from build123d import *

# Parameters (mm, degrees)
F0_W     = 20.141244
F0_H     = 20.141244
F0_R     = 8
F1_DEPTH = 5
F0_R_2   = 6.15
F2_DEPTH = 40
F3_DEPTH = 3


with BuildPart() as f1:
    # F0 (on Top) → F1 (new body)
    with BuildSketch(Plane.XY):
        Rectangle(F0_W, F0_H)
        Circle(F0_R, mode=Mode.SUBTRACT)
    extrude(amount=F1_DEPTH)

    # F0 (on Top) → F2 (join)
    with BuildSketch(Plane.XY):
        Circle(F0_R)
        Circle(F0_R_2, mode=Mode.SUBTRACT)
    extrude(amount=F2_DEPTH)

    # F0 (on Top) → F3 (join)
    with BuildSketch(Plane.XY):
        Circle(F0_R_2)
    extrude(amount=F3_DEPTH)


solid = f1.part
Work out the finished part from the listing and answer in its coordinate system (mm). A direction names the side the tool comes from. Give positions to 0.01 mm unless a question says otherwise; leave off trailing zeros. Order: outer loops, then holes, each group sorted by start corner. A loop starts at its lowest first (then second) coordinate and runs counter-clockwise, first axis right, second up. Notation, with made-up numbers: (79, 47.25) -> (91, 47.25) arc R27 cw to (91, 67.25) -> close; hole circle Ø5 at (46, 42.25). An arc over 180 degrees is marked (long way). Answer as a JSON object with one key per item and string values. Group by question number.
1. A tool of negligible diameter and unlimited length cuts with its end or side. For faces 4 (the flat face through (0, -10.071, 2)), 5 (the flat face through (-5, 7, 5)), from which of +Z, -Z, +X, -X, +Y, -Y can it reach the whole face along a straight path? Write none if from no direction.
2. Section C-C on z = 15 is taken. Determine the outline of the cut face in (x, y), plus the area to 3 significant figures.
3. Flat-ended cylindrical pins translate along their axes: pin 1 Ø7.5 at (x, y) = (0, 0) entering from +Z; pin 2 Ø1.5 at (y, z) = (0.5, 19.5) entering from +X; pin 3 Ø3 at (y, z) = (3.5, 29.5) entering from -X. Find the tip coordinate at first contact, or state that the pin passes through.
4. Section D-D on y = 7 is taken. Determine the outline of the cut face in (x, z).
5. Section A-A on y = 0 is taken. Determine the outline of the cut face in (x, z), plus the area to 3 significant figures.
6. Consider line 1 along Y through (x, z) = (0, 13); line 2 along Z through (x, y) = (-7.75, -8.5); line 3 along Z through (x, y) = (1, 2.75). Determine where each line is inside the solid, lowest interval first. Write a range as [from, to].
7. The mould has two halves that part along Y. Classify faces 1 (the cylindrical face through (-1.333, -6.004, 21.241)), 2 (the cylindrical face through (-1.73, -7.81, 22.26)), 3 (the flat face through (-2, -6, 40)): released by +Y, released by -Y, zero draft, split by the parting line, or undercut.
Result sheet:
{
 "1": {"face 4": "+Z, -Z, +X, -X, -Y", "face 5": "+Z"},
 "2": {"outline": "circle Ø16 at (0, 0); hole circle Ø12.3 at (0, 0)", "area": "82.2 mm^2"},
 "3": {"pin 1": "stops at z = 3", "pin 2": "stops at x = 8", "pin 3": "stops at x = -7.75"},
 "4": {"outline": "(-10.07, 0) -> (10.07, 0) -> (10.07, 5) -> (3.87, 5) -> (3.87, 40) -> (-3.87, 40) -> (-3.87, 5) -> (-10.07, 5) -> close"},
 "5": {"outline": "(-10.07, 0) -> (10.07, 0) -> (10.07, 5) -> (8, 5) -> (8, 40) -> (6.15, 40) -> (6.15, 3) -> (-6.15, 3) -> (-6.15, 40) -> (-8, 40) -> (-8, 5) -> (-10.07, 5) -> close", "area": "206 mm^2"},
 "6": {"line 1": "y = [-8, -6.15], [6.15, 8]", "line 2": "z = [0, 5]", "line 3": "z = [0, 3]"},
 "7": {"face 1": "undercut", "face 2": "split by the parting line", "face 3": "zero draft"}
}
